from build123d import *

# Parameters (mm, degrees)
SKETCH002_R     = 0.425
PAD001_DEPTH    = 12.4
CHAMFER001_SIZE = 0.4
SKETCH003_R     = 0.7
POCKET_DEPTH    = 10.401
CHAMFER_SIZE    = 0.265
SKETCH004_R     = 2.45
POCKET001_DEPTH = 4
CHAMFER002_SIZE = 0.4
FILLET_R        = 0.4


with BuildPart() as part:
    # Sketch002 → Pad001 (new body)
    with BuildSketch(Plane.XY):
        with BuildLine():
            ThreePointArc((-1.015, 7.06), (-3.46011, 5.951013), (-4.236546, 3.380883))
            Line((-4.236546, 3.380883), (-3.221546, -4.239117))
            ThreePointArc((-3.221546, -4.239117), (0, -7.06), (3.221546, -4.239117))
            Line((4.236546, 3.380883), (3.221546, -4.239117))
            ThreePointArc((4.236546, 3.380883), (3.46011, 5.951013), (1.015, 7.06))
            Line((-1.015, 7.06), (1.015, 7.06))
        make_face()
        with Locations((-1.015, 3.81)):
            Circle(SKETCH002_R, mode=Mode.SUBTRACT)
        with Locations((1.015, 3.81)):
            Circle(SKETCH002_R, mode=Mode.SUBTRACT)
        with Locations((0, -3.81)):
            Circle(SKETCH002_R, mode=Mode.SUBTRACT)
    extrude(amount=PAD001_DEPTH)

    # Chamfer001
    chamfer001_edges = [part.edges().sort_by_distance(p)[0] for p in [
        (-1.44, 3.81, 12.4),
        (0.59, 3.81, 12.4),
        (-0.425, -3.81, 12.4),
    ]]
    chamfer(chamfer001_edges, length=CHAMFER001_SIZE)

    # Sketch003 → Pocket (cut, through all)
    with BuildSketch(Plane.XY.offset(10.4)):
        with Locations((0, -3.81)):
            Circle(SKETCH003_R)
        with BuildLine():
            ThreePointArc((-1.015, 4.51), (-1.715, 3.81), (-1.015, 3.11))
            Line((-1.015, 3.11), (1.015, 3.11))
            ThreePointArc((1.015, 3.11), (1.715, 3.81), (1.015, 4.51))
            Line((-1.015, 4.51), (1.015, 4.51))
        make_face()
    extrude(amount=-POCKET_DEPTH, mode=Mode.SUBTRACT)

    # Chamfer
    chamfer_edges = [part.edges().sort_by_distance(p)[0] for p in [
        (1.715, 3.81, 10.4),
        (-0.7, -3.81, 10.4),
    ]]
    chamfer(chamfer_edges, length=CHAMFER_SIZE)

    # Sketch004 → Pocket001 (cut)
    with BuildSketch(Plane.XY.offset(12.4)):
        with Locations((0, -3.81)):
            Circle(SKETCH004_R)
        with BuildLine():
            ThreePointArc((2.089221, -3.5975), (0, -1.71), (-2.089221, -3.5975))
            Line((-2.089221, -3.5975), (2.089221, -3.5975))
        make_face(mode=Mode.SUBTRACT)
        with BuildLine():
            ThreePointArc((-2.089221, -4.0225), (0, -5.91), (2.089221, -4.0225))
            Line((-2.089221, -4.0225), (2.089221, -4.0225))
        make_face(mode=Mode.SUBTRACT)
        with BuildLine():
            ThreePointArc((-1.015, 6.26), (-3.465, 3.81), (-1.015, 1.36))
            Line((-1.015, 1.36), (1.015, 1.36))
            ThreePointArc((1.015, 1.36), (3.465, 3.81), (1.015, 6.26))
            Line((-1.015, 6.26), (1.015, 6.26))
        make_face()
        with BuildLine():
            Line((-1.015, 1.71), (1.015, 1.71))
            ThreePointArc((1.015, 1.71), (2.422793, 2.251754), (3.104225, 3.5975))
            Line((-3.104232, 3.5975), (3.104225, 3.5975))
            ThreePointArc((-3.104232, 3.5975), (-2.422798, 2.251752), (-1.015, 1.71))
        make_face(mode=Mode.SUBTRACT)
        with BuildLine():
            Line((-1.015, 5.91), (1.015, 5.91))
            ThreePointArc((3.104225, 4.0225), (2.422793, 5.368246), (1.015, 5.91))
            Line((-3.104232, 4.0225), (3.104225, 4.0225))
            ThreePointArc((-1.015, 5.91), (-2.422798, 5.368248), (-3.104232, 4.0225))
        make_face(mode=Mode.SUBTRACT)
    extrude(amount=-POCKET001_DEPTH, mode=Mode.SUBTRACT)

    # Chamfer002
    chamfer002_edges = [part.edges().sort_by_distance(p)[0] for p in [
        (-2.458197, 4.0225, 12.4),
        (0, 4.0225, 12.4),
        (2.458194, 4.0225, 12.4),
        (2.422793, 5.368246, 12.4),
        (2.422793, 2.251754, 12.4),
        (2.458194, 3.5975, 12.4),
        (0, 3.5975, 12.4),
        (-2.458197, 3.5975, 12.4),
        (-1.443192, -3.5975, 12.4),
        (1.443192, -3.5975, 12.4),
        (0, -1.71, 12.4),
        (1.443192, -4.0225, 12.4),
        (-1.443192, -4.0225, 12.4),
        (0, -5.91, 12.4),
        (3.46011, 5.951013, 0),
        (3.729046, -0.429117, 0),
        (0, 7.06, 0),
        (0, -7.06, 0),
        (-3.46011, 5.951013, 0),
        (-3.729046, -0.429117, 0),
        (-0.7, -3.81, 0),
        (-1.715, 3.81, 0),
        (0, 3.11, 0),
        (1.715, 3.81, 0),
        (0, 4.51, 0),
        (0, -7.06, 12.4),
    ]]
    chamfer(chamfer002_edges, length=CHAMFER002_SIZE)

    # Fillet
    fillet_edges = [part.edges().sort_by_distance(p)[0] for p in [
        (3.104225, 4.0225, 10.2),
        (-3.104232, 4.0225, 10.2),
        (-3.104232, 3.5975, 10.2),
        (-2.089221, -3.5975, 10.2),
        (-2.089221, -4.0225, 10.2),
        (3.104225, 3.5975, 10.2),
        (2.089221, -4.0225, 10.2),
        (2.089221, -3.5975, 10.2),
    ]]
    fillet(fillet_edges, radius=FILLET_R)


solid = part.part
Here's how the part is built. I have some questions about the finished solid (model axes, mm). A direction names the side the tool comes from. Round coordinates to 2 decimals unless told otherwise and drop trailing zeros. Write each loop counter-clockwise with the first axis right and the second up, starting at its lowest first coordinate (ties: lowest second). Pieces come first, ordered by that corner, then holes. Notation, with made-up numbers: (61.25, 29.25) -> (77.25, 29.25) arc R13 ccw to (77.25, 40.25) -> close; hole circle Ø11 at (-8.5, 72). An arc over 180 degrees is marked (long way). One line per item, written item: value.
1) I'm going to push flat-ended pins straight in: pin 1 Ø3 at (y, z) = (-3.5, 2) entering from +X; pin 2 Ø4 at (x, y) = (1, 4) entering from +Z; pin 3 Ø1.5 at (y, z) = (2, 7) entering from +X; pin 4 Ø1 at (y, z) = (5.5, 5.5) entering from -X. Where does each tip first touch, or does it pass through?
Filled sheet:
pin 1: stops at x = 3.52
pin 2: stops at z = 12.4
pin 3: stops at x = 4.15
pin 4: stops at x = -4.04
2) We'd pull the mould along X, two halves only. Please class faces 1 (the face through (-3.221, 5.789, 0.114)), 2 (the face through (-0.07, -7.06, 6.12)), 3 (the face through (1, -4.022, 10)), 4 (the face through (0.03, -2, 12.29)): released by +X, released by -X, zero draft, split by the parting line, or undercut.
Filled sheet:
face 1: released by -X
face 2: split by the parting line
face 3: undercut
face 4: undercut
3) If I drill on line 1 (Y direction, x = 0, z = 3.25); line 2 (Y direction, x = 0.25, z = 1.25); line 3 (X direction, y = -3.81, z = 6.25), over which ranges is the centre line in solid material (lowest first)? Write a range as [from, to].
Filled sheet:
line 1: y = [-7.06, -4.51], [-3.11, 3.11], [4.51, 7.06]
line 2: y = [-7.05, -4.46], [-3.16, 3.11], [4.51, 7.06]
line 3: x = [-3.28, -0.7], [0.7, 3.28]
4) Suppose I cut it at D-D on y = -3.81. List the corners of the cut face in (x, z) for me, plus the area to 3 significant figures.
Filled sheet:
outline: (-3.28, 0.4) -> (-2.88, 0) -> (-1.1, 0) -> (-0.7, 0.4) -> (-0.7, 8.4) -> (-2.45, 8.4) -> (-2.45, 12.4) -> (-2.88, 12.4) -> (-3.28, 12) -> close; (0.7, 0.4) -> (1.1, 0) -> (2.88, 0) -> (3.28, 0.4) -> (3.28, 12) -> (2.88, 12.4) -> (2.45, 12.4) -> (2.45, 8.4) -> (0.7, 8.4) -> close
area: 49.5 mm2
5) Suppose I cut it at B-B on y = 3.81. List the corners of the cut face in (x, z) for me (3 decimals), plus the area to 3 significant figures.
Filled sheet:
outline: (-4.265, 0.4) -> (-3.865, 0) -> (-2.115, 0) -> (-1.715, 0.4) -> (-1.715, 8.4) -> (-3.465, 8.4) -> (-3.465, 12.4) -> (-3.865, 12.4) -> (-4.265, 12) -> close; (1.715, 0.4) -> (2.115, 0) -> (3.865, 0) -> (4.265, 0.4) -> (4.265, 12) -> (3.865, 12.4) -> (3.465, 12.4) -> (3.465, 8.4) -> (1.715, 8.4) -> close
area: 48.8 mm2
6) Suppose I cut it at C-C on x = 0. Give the number of separate pieces and of enclosed holes in the cut face, plus the area to 3 significant figures.
Filled sheet:
separate pieces: 3
enclosed holes: 0
area: 137 mm2
7) Suppose I cut it at A-A on z = 4.5. List the corners of the cut face in (x, y) for me (3 decimals).
Filled sheet:
outline: (-4.237, 3.381) -> (-3.222, -4.239) arc R3.25 ccw to (3.222, -4.239) -> (4.237, 3.381) arc R3.25 ccw to (1.015, 7.06) -> (-1.015, 7.06) arc R3.25 ccw to start; hole (-1.015, 3.11) -> (1.015, 3.11) arc R0.7 ccw to (1.015, 4.51) -> (-1.015, 4.51) arc R0.7 ccw to start; hole circle Ø1.4 at (0, -3.81)
8) For faces 5 (the face through (-3.54, -0.35, 12.2)), 6 (the face through (-1.823, 3.828, 0.292)), 7 (the face through (0.04, -1.71, 10.23)), which set-ups out of +Z, -Z, +X, -X, +Y, -Y let a thin tool reach every point of the face, with its end or its side?
Filled sheet:
face 5: +Z, -X, -Y
face 6: -Z
face 7: +Z
